Part model, mm, in its own coordinate system. A direction names the side the tool comes from. Coordinates: 2 decimals unless noted, no trailing zeros. Loops run counter-clockwise (first coordinate to the right, second up) from the corner with the lowest first, then second, coordinate; pieces in that order, holes last. Notation, with made-up numbers: (10, 38.25) - (51, 38.25) arc R29 ccw to (51, 62.25) - close; hole circle Ø2 at (70, 56.5). An arc over 180 degrees is marked (long way). One line per question, with ' | ' between items. Start each with the question number.
from build123d import *

# Parameters (mm, degrees)
SKETCH030_W        = 119.5
SKETCH030_H        = 76
SKETCH030_R        = 1.4
PAD009_DEPTH       = 15
SKETCH031_W        = 119.5
SKETCH031_H        = 76
PAD010_DEPTH       = 7
SKETCH032_W        = 12
SKETCH032_H        = 11
POCKET011_DEPTH    = 7
HOLE_D             = 3.4
HOLE_CBORE_D       = 6.1
HOLE_CBORE_DEPTH   = 3.4
PAD013_DEPTH       = 22
CHAMFER001_1_ANGLE = 5
CHAMFER001_1_SIZE  = 21
CHAMFER001_2_ANGLE = 5
CHAMFER001_2_SIZE  = 21
CHAMFER003_SIZE    = 3
CHAMFER004_SIZE    = 1
CHAMFER005_SIZE    = 1


with BuildPart() as part:
    # Sketch030 (on Face1 of Binder008) → Pad009 (new body)
    with BuildSketch(Plane(origin=(0, 0, -1.6), x_dir=(1, 0, 0), z_dir=(0, 0, -1))):
        with Locations((50.75, 29)):
            Rectangle(SKETCH030_W, SKETCH030_H)
        with Locations((3.5, 54.5)):
            Circle(SKETCH030_R, mode=Mode.SUBTRACT)
        with Locations((98, 54.5)):
            Circle(SKETCH030_R, mode=Mode.SUBTRACT)
        with Locations((98, 3.5)):
            Circle(SKETCH030_R, mode=Mode.SUBTRACT)
        with Locations((3.5, 3.5)):
            Circle(SKETCH030_R, mode=Mode.SUBTRACT)
        Polygon((-2, 52), (-2, 6), (6, 6), (6, -2), (95.5, -2), (95.5, 6), (103.5, 6), (103.5, 52), (95.5, 52), (95.5, 60), (6, 60), (6, 52), align=None, mode=Mode.SUBTRACT)
    extrude(amount=PAD009_DEPTH)

    # Sketch031 (on Face22 of Pad009) → Pad010 (join)
    with BuildSketch(Plane(origin=(0, 0, -16.6), x_dir=(1, 0, 0), z_dir=(0, 0, -1))):
        with Locations((50.75, 29)):
            Rectangle(SKETCH031_W, SKETCH031_H)
    extrude(amount=PAD010_DEPTH)

    # Sketch032 (on Face26 of Pad010) → Pocket011 (cut)
    with BuildSketch(Plane(origin=(0, 9, 0), x_dir=(-1, 0, 0), z_dir=(0, 1, 0))):
        with Locations((-19, -7.1)):
            Rectangle(SKETCH032_W, SKETCH032_H)
    extrude(amount=-POCKET011_DEPTH, mode=Mode.SUBTRACT)

    # Hole (through all)
    with Locations(Plane(origin=(0, 0, -23.6), x_dir=(1, 0, 0), z_dir=(0, 0, -1))):
        with Locations((-2, 60), (103.5, 60), (103.5, -2), (-2, -2)):
            CounterBoreHole(HOLE_D / 2, HOLE_CBORE_D / 2, HOLE_CBORE_DEPTH)

    # Sketch038 (on Face1 of Hole) → Pad013 (join)
    with BuildSketch(Plane.XY.offset(-1.6)):
        Polygon((81.571463, 9), (59.171468, 9), (56.284717, 14), (84.458214, 14), align=None)
    extrude(amount=-PAD013_DEPTH)

    # Chamfer001 1
    chamfer001_1_edges = [part.edges().sort_by_distance(p)[0] for p in [
        (83.014838, 11.5, -1.6),
    ]]
    chamfer001_1_side = part.faces().sort_by_distance((83.014838, 11.5, -12.6))[0]
    chamfer(chamfer001_1_edges, length=CHAMFER001_1_SIZE, angle=CHAMFER001_1_ANGLE, reference=chamfer001_1_side)

    # Chamfer001 2
    chamfer001_2_edges = [part.edges().sort_by_distance(p)[0] for p in [
        (57.728092, 11.5, -1.6),
    ]]
    chamfer001_2_side = part.faces().sort_by_distance((57.728092, 11.5, -12.6))[0]
    chamfer(chamfer001_2_edges, length=CHAMFER001_2_SIZE, angle=CHAMFER001_2_ANGLE, reference=chamfer001_2_side)

    # Chamfer003
    chamfer003_edges = [part.edges().sort_by_distance(p)[0] for p in [
        (110.5, 9, -12.6),
        (110.5, -29, -23.6),
        (110.5, -67, -12.6),
        (50.75, -67, -23.6),
        (-9, 9, -12.6),
        (-9, -29, -23.6),
        (-9, -67, -12.6),
    ]]
    chamfer(chamfer003_edges, length=CHAMFER003_SIZE)

    # Chamfer004
    chamfer004_edges = [part.edges().sort_by_distance(p)[0] for p in [
        (26.585734, 9, -23.6),
        (94.535731, 9, -23.6),
    ]]
    chamfer(chamfer004_edges, length=CHAMFER004_SIZE)

    # Chamfer005
    chamfer005_edges = [part.edges().sort_by_distance(p)[0] for p in [
        (13, 9, -7.1),
        (19, 9, -12.6),
        (25, 9, -7.1),
    ]]
    chamfer(chamfer005_edges, length=CHAMFER005_SIZE)


solid = part.part
1) Band-saw the part on C-C on x = 36. List the corners of the cut face in (y, z), then the cut area to 3 significant figures.
2) Band-saw the part on A-A on x = 98. List the corners of the cut face in (y, z).
3) Tool access for faces 4 (the flat face through (50, -67, -11)), 5 (the flat face through (58.8, 11.5, -12)), 6 (the cylindrical face through (3.32, -55.89, -8.99)), 7 (the flat face through (-0.69, 3.31, -20.2)): list every direction of +Z, -Z, +X, -X, +Y, -Y with a clear straight run to the whole face (end or side of a thin tool).
4) Band-saw the part on D-D on y = -34.5. List the corners of the cut face in (x, z).
5) Pin check, flat tips, straight feed: pin 1 Ø5 at (x, y) = (-1, 3) entering from -Z; pin 2 Ø3 at (x, y) = (18.5, 5.5) entering from +Z; pin 3 Ø3 at (x, y) = (-1, -60) entering from -Z; pin 4 Ø9 at (x, z) = (2, -8.5) entering from +Y. Stop position of each tip, or through.
6) Wall check: line 1 along X through (y, z) = (-3.5, -10.25); line 2 along Y through (x, z) = (16, -14.5); line 3 along Y through (x, z) = (58.5, -12.75). Give the ranges that are in metal, low to high. Write a range as [from, to].
7) Band-saw the part on B-B on y = -54.5. List the corners of the cut face in (x, z).
8) Mould opens along Y. For faces 1 (the flat face through (-8, 7, -12)), 2 (the flat face through (13, 5, -7)), 3 (the cylindrical face through (4.15, -2.26, -8.99)) say: +Y half, -Y half, draft (parallel to the pull), parting line (faces both ways), or undercut.
Values found:
1) outline: (-67, -20.6) - (-64, -23.6) - (8, -23.6) - (9, -22.6) - (9, -1.6) - (2, -1.6) - (2, -16.6) - (-60, -16.6) - (-60, -1.6) - (-67, -1.6) - close | area: 737 mm²
2) outline: (-67, -20.6) - (-64, -23.6) - (8, -23.6) - (9, -22.6) - (9, -1.6) - (-2.1, -1.6) - (-2.1, -16.6) - (-4.9, -16.6) - (-4.9, -1.6) - (-6, -1.6) - (-6, -16.6) - (-52, -16.6) - (-52, -1.6) - (-53.1, -1.6) - (-53.1, -16.6) - (-55.9, -16.6) - (-55.9, -1.6) - (-67, -1.6) - close
3) face 4: +Z, -Z, +X, -X, -Y | face 5: +Z, -X | face 6: +Z | face 7: -Z
4) outline: (-9, -20.6) - (-6, -23.6) - (107.5, -23.6) - (110.5, -20.6) - (110.5, -1.6) - (103.5, -1.6) - (103.5, -16.6) - (-2, -16.6) - (-2, -1.6) - (-9, -1.6) - close
5) pin 1: z = -23.6 | pin 2: z = -12.6 | pin 3: z = -20.2 | pin 4: y = 9
6) line 1: [-9, 2.1], [4.9, 6], [95.5, 96.6], [99.4, 110.5] | line 2: [-67, -60], [2, 9] | line 3: [-67, -60], [2, 9], [11.89, 14]
7) outline: (-9, -20.6) - (-6, -23.6) - (107.5, -23.6) - (110.5, -20.6) - (110.5, -1.6) - (99.4, -1.6) - (99.4, -16.6) - (96.6, -16.6) - (96.6, -1.6) - (95.5, -1.6) - (95.5, -16.6) - (6, -16.6) - (6, -1.6) - (4.9, -1.6) - (4.9, -16.6) - (2.1, -16.6) - (2.1, -1.6) - (-9, -1.6) - close
8) face 1: +Y half | face 2: draft | face 3: undercut
